Part model, mm, in its own coordinate system. A direction names the side the tool comes from. Round coordinates to 2 decimals unless told otherwise and drop trailing zeros. Order: outer loops, then holes, each group sorted by start corner. A loop starts at its lowest first (then second) coordinate and runs counter-clockwise, first axis right, second up. Notation, with made-up numbers: (-30, 82.25) -> (9, 82.25) arc R19 cw to (9, 108.25) -> close; hole circle Ø7 at (64, -40). An arc over 180 degrees is marked (long way). Answer as a JSON object with one key per item and string values. Group by question number.
```python
from build123d import *

# Parameters (mm, degrees)
SKETCH1_W           = 6.6675
SKETCH1_H           = 25.4
SKETCH2_W           = 3.302
SKETCH2_H           = 62.357
BOSS_EXTRUDE1_DEPTH = 25.4
CIRPATTERN1_COUNT   = 12
FILLET1_R           = 2.54
SKETCH4_R           = 5.08
SKETCH4_R_2         = 1.5875
BOSS_EXTRUDE2_DEPTH = 25.4
SKETCH5_R           = 1.5875
CUT_EXTRUDE2_DEPTH  = 25.4
CIRPATTERN2_COUNT   = 4


with BuildPart() as part:
    # Sketch1 → Revolve1 (revolve)
    with BuildSketch(Plane.XY, mode=Mode.PRIVATE) as revolve1_sk:
        with Locations((9.68375, 0)):
            Rectangle(SKETCH1_W, SKETCH1_H)
    revolve(revolve1_sk.sketch.rotate(Axis((0, 37.278132, 0), (0, -1, 0)), 90), axis=Axis((0, 37.278132, 0), (0, -1, 0)))

    # Sketch2 → Boss-Extrude1 (add)
    with BuildSketch(Plane(origin=(0, 12.7, 0), x_dir=(1, 0, 0), z_dir=(0, 1, 0))):
        with Locations((0, -41.3385)):
            Rectangle(SKETCH2_W, SKETCH2_H)
    boss_extrude1 = extrude(amount=-BOSS_EXTRUDE1_DEPTH)

    # CirPattern1: Boss-Extrude1 ×12 about axis
    cirpattern1_axis = Axis((0, 0, 0), (0, 1, 0))
    for i in range(1, CIRPATTERN1_COUNT):
        add(boss_extrude1.rotate(cirpattern1_axis, i * 360 / CIRPATTERN1_COUNT))

    # Fillet1
    # the kernel refuses this fillet: 2.54 mm, written as the material it adds along each edge
    with BuildSketch(Plane(origin=(12.007947359, 12.7, -5.026381051), x_dir=(0.8660254037844386, 0, -0.5000000000000003), z_dir=(0, -1, 0)), Plane(origin=(7.885996935, 12.7, -10.356947359), x_dir=(0.5000000000000001, 0, -0.8660254037844385), z_dir=(0, -1, 0))) as fillet1_piece_1:
        with BuildLine():
            CenterArc((2.069989159, 2.54), FILLET1_R, 195.62783797, 74.37216203)
            ThreePointArc((-0.3761116, 1.855755102), (-0.154269512, 0.934725122), (0, 0))
            Line((0, 0), (2.069989159, 0))
        make_face()
    extrude(amount=25.4)
    with BuildSketch(Plane(origin=(10.356947359, 12.7, -7.885996935), x_dir=(-0.6620593723913752, 0, -0.7494513909712479), z_dir=(0, -1, 0)), Plane(origin=(5.026381051, 12.7, -12.007947359), x_dir=(-0.9480859307901371, 0, -0.31801425728699545), z_dir=(0, -1, 0))) as fillet1_piece_2:
        with BuildLine():
            CenterArc((2.078215675, 2.533273519), FILLET1_R, 191.457121991, 74.37216203)
            Line((-0.411171344, 2.028741788), (0, 0))
            ThreePointArc((0, 0), (0.946742697, 0.034473214), (1.893485393, 0))
        make_face()
    extrude(amount=25.4)

    # Sketch4 → Boss-Extrude2 (add)
    with BuildSketch(Plane(origin=(0, 12.7, 0), x_dir=(1, 0, 0), z_dir=(0, 1, 0))):
        with Locations((0, 63.5)):
            Circle(SKETCH4_R)
        with Locations((0, 63.5)):
            Circle(SKETCH4_R_2, mode=Mode.SUBTRACT)
    boss_extrude2 = extrude(amount=-BOSS_EXTRUDE2_DEPTH)

    # Sketch5 → Cut-Extrude2 (cut)
    with BuildSketch(Plane(origin=(0, 12.7, 0), x_dir=(1, 0, 0), z_dir=(0, 1, 0))):
        with Locations(Location((0, 63.5, 0), (0, 0, 270))):
            Circle(SKETCH5_R)
    cut_extrude2 = extrude(amount=-CUT_EXTRUDE2_DEPTH, mode=Mode.SUBTRACT)

    # CirPattern2: Boss-Extrude2, Cut-Extrude2 ×4 about axis
    cirpattern2_axis = Axis((0, 0, 0), (0, 1, 0))
    add([boss_extrude2.rotate(cirpattern2_axis, i * 360 / CIRPATTERN2_COUNT) for i in range(1, CIRPATTERN2_COUNT)])
    add([cut_extrude2.rotate(cirpattern2_axis, i * 360 / CIRPATTERN2_COUNT) for i in range(1, CIRPATTERN2_COUNT)], mode=Mode.SUBTRACT)


solid = part.part
```
Q1. Drop flat-ended pins along their axis: pin 1 Ø2.5 at (x, z) = (0, -63.5) entering from +Y; pin 2 Ø4.5 at (y, z) = (-3, -69.5) entering from +X; pin 3 Ø4.5 at (x, y) = (-69.5, 3) entering from +Z; pin 4 Ø4.5 at (x, y) = (70, -2.5) entering from -Z. Give the stop position or say it passes through.
Q2. Band-saw the part on D-D (y = 7). Count the separate pieces of the cut face and the enclosed holes in it, plus the area to 3 significant figures.
Q3. Band-saw the part on B-B (x = 56). List the corners of the cut face in (y, z), plus the area to 3 significant figures.
Q4. Two-plate mould, pull along X, no slides. Class faces 5 (the flat face through (-72.517, 0, 0)), 6 (the flat face through (-20.136, 0.178, 38.179)), 7 (the flat face through (38.179, 0.178, 20.136)): +X half, -X half, draft (parallel to the pull), parting line (faces both ways), or undercut.
Q5. Which spindle directions (+Z, -Z, +X, -X, +Y, -Y) get a long thin tool onto all of the face, cutting with end or side? Do faces 1 (the flat face through (-36, 0, -1.651)), 2 (the flat face through (-38.179, 0.178, -20.136)), 3 (the flat face through (-6, -12.7, 6)), 4 (the flat face through (-1.651, 0, -70)). Say none if no direction does.
Q6. Band-saw the part on A-A (z = 21). List the corners of the cut face in (x, y), plus the area to 3 significant figures.
Q7. Band-saw the part on C-C (z = 57). List the corners of the cut face in (x, y).
Q8. Wall check: line 1 (X direction, y = 3, z = 15); line 2 (X direction, y = -5.5, z = -63.5); line 3 (Z direction, x = 2, y = -2.25). Give the ranges that are in metal, low to high. Write a range as [from, to].
Completed:
{
 "1": {"pin 1": "through", "pin 2": "x = 3.43", "pin 3": "z = 3.43", "pin 4": "z = -2.78"},
 "2": {"separate pieces": "1", "enclosed holes": "5", "area": "2,930 mm2"},
 "3": {"outline": "(-12.7, -34.24) -> (12.7, -34.24) -> (12.7, -30.43) -> (-12.7, -30.43) -> close; (-12.7, -1.65) -> (12.7, -1.65) -> (12.7, 1.65) -> (-12.7, 1.65) -> close; (-12.7, 30.43) -> (12.7, 30.43) -> (12.7, 34.24) -> (-12.7, 34.24) -> close", "area": "278 mm2"},
 "4": {"face 5": "-X half", "face 6": "undercut", "face 7": "+X half"},
 "5": {"face 1": "+Y, -Y", "face 2": "-X, +Y, -Y", "face 3": "+Z, -Z, +X, -X, -Y", "face 4": "-Z, -X, +Y, -Y"},
 "6": {"outline": "(-39.68, -12.7) -> (-33.07, -12.7) -> (-33.07, 12.7) -> (-39.68, 12.7) -> close; (-14.03, -12.7) -> (-10.22, -12.7) -> (-10.22, 12.7) -> (-14.03, 12.7) -> close; (-1.65, -12.7) -> (1.65, -12.7) -> (1.65, 12.7) -> (-1.65, 12.7) -> close; (10.22, -12.7) -> (14.03, -12.7) -> (14.03, 12.7) -> (10.22, 12.7) -> close; (33.07, -12.7) -> (39.68, -12.7) -> (39.68, 12.7) -> (33.07, 12.7) -> close", "area": "613 mm2"},
 "7": {"outline": "(-34.82, -12.7) -> (-31, -12.7) -> (-31, 12.7) -> (-34.82, 12.7) -> close; (-1.65, -12.7) -> (1.65, -12.7) -> (1.65, 12.7) -> (-1.65, 12.7) -> close; (31, -12.7) -> (34.82, -12.7) -> (34.82, 12.7) -> (31, 12.7) -> close"},
 "8": {"line 1": "[-29.28, -22.68], [-10.57, -6.75], [-1.65, 1.65], [6.75, 10.57], [22.68, 29.28]", "line 2": "[-35.05, -34.76], [-5.08, -1.59], [1.59, 5.08], [34.76, 35.05]", "line 3": "[-68.17, -58.83], [-12.86, -6.03], [6.03, 12.86], [58.83, 68.17]"}
}
